Could you check a few things on this drawing? It's one solid part, dimensions in mm from its lowest x, y, z. Coordinates: 2 decimals unless noted, no trailing zeros. Write each loop counter-clockwise with the first axis right and the second up, starting at its lowest first coordinate (ties: lowest second). Pieces come first, ordered by that corner, then holes.
Item 1: I want a section at A-A (z = 0.6). Please give me the cut outline in (x, y), and give its area (3 significant figures).
Item 2: I'm going to push flat-ended pins straight in: P1, Ø0.6, axis at y = 1.5, z = 2, coming from the -X side; P2, Ø3, axis at x = 9.5, y = 9.5, coming from the -Z side; P3, Ø1, axis at y = 44, z = 1, coming from the +X side. Where does each tip first touch, or does it pass through?
Item 3: Please list where these lines run through material, in increasing order: line 1 (Y direction, x = 13.75, z = 2.6); line 2 (Y direction, x = 3.75, z = 2.55); line 3 (X direction, y = 5, z = 1.5).
Item 4: I want a section at B-B (x = 1). Please give me the cut outline in (y, z).
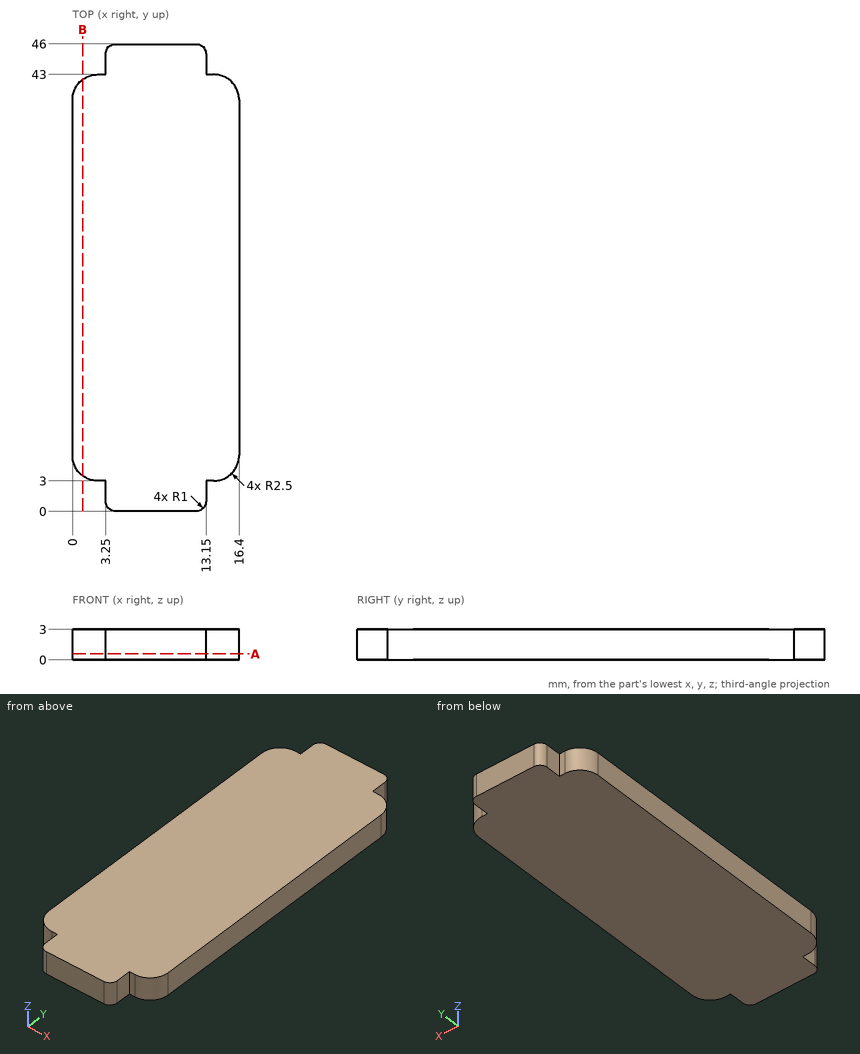
Answer:
1. outline: (0, 5.5) arc R2.5 ccw to (2.5, 3) - (3.25, 3) - (3.25, 1) arc R1 ccw to (4.25, 0) - (12.15, 0) arc R1 ccw to (13.15, 1) - (13.15, 3) - (13.9, 3) arc R2.5 ccw to (16.4, 5.5) - (16.4, 40.5) arc R2.5 ccw to (13.9, 43) - (13.15, 43) - (13.15, 45) arc R1 ccw to (12.15, 46) - (4.25, 46) arc R1 ccw to (3.25, 45) - (3.25, 43) - (2.5, 43) arc R2.5 ccw to (0, 40.5) - close
1. area: 709 mm2
2. P1: stops at x = 3.25
2. P2: stops at z = 0
2. P3: stops at x = 13.15
3. line 1: y = 3 to 43
3. line 2: y = 0.13 to 45.87
3. line 3: x = 0.05 to 16.35
4. outline: (3.5, 0) - (42.5, 0) - (42.5, 3) - (3.5, 3) - close
